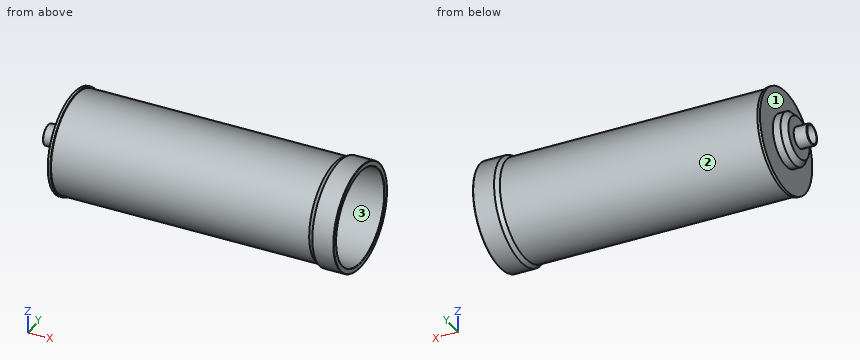
Autodesk Inventor part; units mm, degrees
ref_plane "Work Plane1" through (404, 0, 0) normal (1, 0, 0) x (0, 0, -1)
ref_plane "YZ Plane" through (0, 0, 0) normal (1, 0, 0) x (0, 1, 0)
ref_plane "XZ Plane" through (0, 0, 0) normal (0, 1, 0) x (-1, 0, 0)
sketch "Sketch3" plane through (0, 0, 0) normal (1, 0, 0) x (0, 1, 0)
  circle A0 centre (0, 0) radius 79
extrude "Extrusion2" add sketch "Sketch3" along normal blind 4
sketch "Sketch4" plane through (4, 0, 0) normal (1, 0, 0) x (0, 0, -1)
  circle A0 centre (0, 0) radius 77
  circle A1 centre (0, 0) radius 73
extrude "Extrusion3" add sketch "Sketch4" along normal blind 400
ref_plane "Work Plane1" through (404, 0, 0) normal (1, 0, 0) x (0, 0, -1)
sketch "Sketch5" plane through (404, 0, 0) normal (1, 0, 0) x (0, 0, -1)
  circle A0 centre (0, 0) radius 81
  circle A1 centre (0, 0) radius 73
extrude "Extrusion4" add sketch "Sketch5" along normal blind 40
chamfer "Chamfer1" distance 4 angle 60 1 edges at (404, 0, 81) measured on face at (404, 0, 78.1669)
sketch "Sketch7" plane through (0, 0, 0) normal (-1, 0, 0) x (0, 0, 1)
  circle A0 centre (0, 0) radius 16
  circle A1 centre (0, 0) radius 40
  circle A2 centre (0, 0) radius 14
extrude "Extrusion5" add sketch "Sketch7" along normal blind 20 contours A1
extrude "Extrusion6" add sketch "Sketch7" along normal blind 40 contours A0
fillet "Fillet1" radius 0.8 1 edges at (-40, 0, -16)
chamfer "Chamfer2" distance 8 angle 45 1 edges at (-20, 0, -40)
fillet "Fillet2" radius 1 2 edges at (444, 0, 81) (444, 0, 73)
extrude "Extrusion7" cut sketch "Sketch7" against normal through all contours A2
sketch "Sketch8" plane through (0, 0, 0) normal (-1, 0, 0) x (0, 0, 1)
  point P0 (0, 0)
properties part number "GuiderTube"
Build history of the part. All positions in model axes, mm. Face numbers are marked on the shaded views. Round coordinates to 2 decimals unless told otherwise and drop trailing zeros. Write each loop counter-clockwise with the first axis right and the second up, starting at its lowest first coordinate (ties: lowest second). Pieces come first, ordered by that corner, then holes. Notation, with made-up numbers: M -28,35 L 29,35 A28 cw 29,68 Z; hole C 65.5,16 d3. An arc over 180 degrees is marked long. Answer in a Markdown table with one row per item.
1. Probe L1, parallel to Y at x = 126.5, z = 0; L2, parallel to X at y = -14, z = -24.5; L3, parallel to X at y = 42, z = -11.5. List the from-to ranges inside material, lowest first. Write a range as [from, to].
Geometry check:
| item | result |
|---|---|
| L1 | [-77, -73], [73, 77] |
| L2 | [-20, 4] |
| L3 | [0, 4] |
2. Saw through at A-A (x = 81). List the corners of the cut face in (y, z), and give its area (3 significant figures).
Geometry check:
| item | result |
|---|---|
| outline | C 0,0 d154; hole C 0,0 d146 |
| area | 1,880 mm2 |
3. Flat gauge pins, fed straight in: P1, Ø12, axis at y = -58, z = 58.5, coming from the +X side; P2, Ø10, axis at x = 196.5, z = -43, coming from the -Y side; P3, Ø10, axis at x = 230, y = -7.5, coming from the -Z side; P4, Ø1.5, axis at x = 61, z = 63, coming from the +Y side. Where does each tip first touch, or does it go through?
Geometry check:
| item | result |
|---|---|
| P1 | x = 444 |
| P2 | y = -66.97 |
| P3 | z = -76.96 |
| P4 | y = 45.32 |
4. Mould opens along Z. For the marked faces 1, 2 and 3 say: +Z half, -Z half, draft (parallel to the pull), parting line (faces both ways), or undercut.
Geometry check:
| item | result |
|---|---|
| face 1 | draft |
| face 2 | parting line |
| face 3 | undercut |
